```python
from build123d import *

# Parameters (mm, degrees)
SKETCH1_R           = 3
BOSS_EXTRUDE1_DEPTH = 30
SKETCH2_R           = 3.420462188
BOSS_EXTRUDE2_DEPTH = 5
CUT_EXTRUDE1_DEPTH  = 4
BOSS_EXTRUDE3_START = 50.360841313
SKETCH4_R           = 3
BOSS_EXTRUDE3_DEPTH = 50.360841313


with BuildPart() as part:
    # Sketch1 → Boss-Extrude1 (new body)
    with BuildSketch(Plane(origin=(0, 0, 0), x_dir=(1, 0, 0), z_dir=(0, 1, 0))):
        with Locations(Location((0, 0, 0), (0, 0, 270))):
            Circle(SKETCH1_R)
    extrude(amount=BOSS_EXTRUDE1_DEPTH)

    # Sketch2 → Boss-Extrude2 (add)
    with BuildSketch(Plane(origin=(0, 30, 0), x_dir=(1, 0, 0), z_dir=(0, 1, 0))):
        with Locations(Location((0, 0, 0), (0, 0, 270))):
            Circle(SKETCH2_R)
    extrude(amount=BOSS_EXTRUDE2_DEPTH)

    # Sketch3 → Cut-Extrude1 (cut)
    with BuildSketch(Plane(origin=(0, 35, 0), x_dir=(1, 0, 0), z_dir=(0, 1, 0))):
        Polygon((-0.25878856, 2.462260088), (-2.261774067, 1.007012576), (-2.002985506, -1.455247511), (0.25878856, -2.462260088), (2.261774067, -1.007012576), (2.002985506, 1.455247511), align=None)
    extrude(amount=-CUT_EXTRUDE1_DEPTH, mode=Mode.SUBTRACT)

    # Sketch4 → Boss-Extrude3 (add)
    with BuildSketch(Plane(origin=(0, 0, 0), x_dir=(-1, 0, 0), z_dir=(0, -1, 0)).offset(BOSS_EXTRUDE3_START)):
        with Locations(Location((0, 0, 0), (0, 0, 90))):
            Circle(SKETCH4_R)
    extrude(amount=-BOSS_EXTRUDE3_DEPTH)


solid = part.part
```
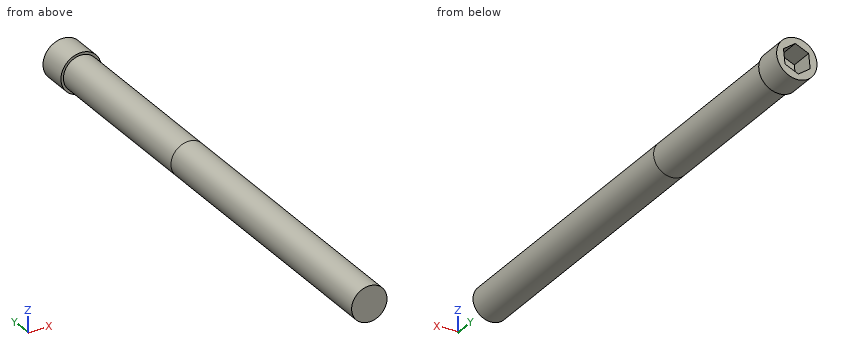
Could you check a few things on this model? Use its own coordinates, in mm. Give positions to 0.01 mm unless a question says otherwise; leave off trailing zeros. Write each loop counter-clockwise with the first axis right and the second up, starting at its lowest first coordinate (ties: lowest second). Pieces come first, ordered by that corner, then holes. Notation, with made-up numbers: (0, -1.75) - (18, -1.75) arc R21 ccw to (18, 14.25) - close; hole circle Ø9 at (69, -38.75). An arc over 180 degrees is marked (long way). One line per item, written item: value. Start each with the question number.
Item 1: Please list where these lines run through material, in increasing order: line 1 (Y direction, x = 1.5, z = 3); line 2 (Y direction, x = 1, z = 0.25); line 3 (Z direction, x = 0.25, y = 16). Write a range as from..to.
Item 2: I'm going to push flat-ended pins straight in: pin 1 (1.5 mm diameter, centred on x = 1, y = 23.5, fed in from +Z); pin 2 (2 mm diameter, centred on y = 20, z = 1.5, fed in from +X); pin 3 (1.4 mm diameter, centred on x = -1, z = -1, fed in from +Y). Where does each tip first touch, or does it pass through?
Item 3: Imagine slicing it at A-A, the plane z = 0. List the corners of the cut face in (x, y) for me.
Item 4: Imagine slicing it at B-B, the plane x = 1.25. List the corners of the cut face in (y, z) for me, and give its area (3 significant figures).
Item 5: Imagine slicing it at C-C, the plane y = 13.5. List the corners of the cut face in (x, z) for me, and give its area (3 significant figures).
Geometry says:
1. line 1: 30..35
1. line 2: -50.36..31
1. line 3: -2.99..2.99
2. pin 1: z = 2.99
2. pin 2: x = 2.96
2. pin 3: y = 31
3. outline: (-3.42, 30) - (-3, 30) - (-3, -50.36) - (3, -50.36) - (3, 30) - (3.42, 30) - (3.42, 35) - (2.16, 35) - (2.16, 31) - (-2.16, 31) - (-2.16, 35) - (-3.42, 35) - close
4. outline: (-50.36, -2.73) - (30, -2.73) - (30, -3.18) - (35, -3.18) - (35, -1.79) - (31, -1.79) - (31, 1.74) - (35, 1.74) - (35, 3.18) - (30, 3.18) - (30, 2.73) - (-50.36, 2.73) - close
4. area: 456 mm^2
5. outline: circle Ø6 at (0, 0)
5. area: 28.3 mm^2
